Source: CAD feature listing. Evaluate the final solid. Frame: model axes, mm. Give positions to 0.01 mm unless a question says otherwise; leave off trailing zeros. Write each loop counter-clockwise with the first axis right and the second up, starting at its lowest first coordinate (ties: lowest second). Pieces come first, ordered by that corner, then holes.
```python
from build123d import *

# Parameters (mm, degrees)
SKETCH1_W           = 5
SKETCH1_H           = 28.000000001
SKETCH1_H_2         = 5
BOSS_EXTRUDE1_DEPTH = 5


with BuildPart() as part:
    # Sketch1 → Boss-Extrude1 (new body)
    with BuildSketch(Plane.XY):
        Polygon((331, 10), (323.5, 10), (323.5, 5), (318.5, 5), (318.5, 10), (2.5, 10), (2.5, 5), (-2.5, 5), (-2.5, 10), (-10, 10), (-10, 2.5), (-5, 2.5), (-5, -2.5), (-10, -2.5), (-10, -227.5), (-5, -227.5), (-5, -232.5), (-10, -232.5), (-10, -240), (-2.5, -240), (-2.5, -235), (2.5, -235), (2.5, -240), (318.5, -240), (318.5, -235), (323.5, -235), (323.5, -240), (331, -240), (331, -232.5), (326, -232.5), (326, -227.5), (331, -227.5), (331, -2.5), (326, -2.5), (326, 2.5), (331, 2.5), align=None)
        with Locations((-5.5, -128.600000001)):
            Rectangle(SKETCH1_W, SKETCH1_H, mode=Mode.SUBTRACT)
        with Locations((326.5, -128.600000001)):
            Rectangle(SKETCH1_W, SKETCH1_H, mode=Mode.SUBTRACT)
        with Locations((313.5, 0)):
            Rectangle(SKETCH1_W, SKETCH1_H_2, mode=Mode.SUBTRACT)
        with Locations((321, -7.5)):
            Rectangle(SKETCH1_W, SKETCH1_H_2, mode=Mode.SUBTRACT)
        with Locations((0, -7.5)):
            Rectangle(SKETCH1_W, SKETCH1_H_2, mode=Mode.SUBTRACT)
        with Locations((7.5, 0)):
            Rectangle(SKETCH1_W, SKETCH1_H_2, mode=Mode.SUBTRACT)
        with Locations((160.5, -122.5)):
            Rectangle(SKETCH1_W, SKETCH1_H_2, mode=Mode.SUBTRACT)
        with Locations((168, -115)):
            Rectangle(SKETCH1_W, SKETCH1_H_2, mode=Mode.SUBTRACT)
        with Locations((153, -115)):
            Rectangle(SKETCH1_W, SKETCH1_H_2, mode=Mode.SUBTRACT)
        with Locations((160.5, -107.5)):
            Rectangle(SKETCH1_W, SKETCH1_H_2, mode=Mode.SUBTRACT)
        with Locations((7.5, -230)):
            Rectangle(SKETCH1_W, SKETCH1_H_2, mode=Mode.SUBTRACT)
        with Locations((0, -222.5)):
            Rectangle(SKETCH1_W, SKETCH1_H_2, mode=Mode.SUBTRACT)
        with Locations((321, -222.5)):
            Rectangle(SKETCH1_W, SKETCH1_H_2, mode=Mode.SUBTRACT)
        with Locations((313.5, -230)):
            Rectangle(SKETCH1_W, SKETCH1_H_2, mode=Mode.SUBTRACT)
    extrude(amount=BOSS_EXTRUDE1_DEPTH)


solid = part.part
```
1. Line query: probe 1 along X at (y, z) = (-136, 0.2); probe 2 along X at (y, z) = (-221, 1.55); probe 3 along X at (y, z) = (-124, 3.6). Output: solid intervals per line, ascending.
2. Pin query (flat end, axial travel): P1, Ø2.5, axis at y = 0.5, z = 1.5, coming from the +X side; P2, Ø2.5, axis at y = -230.5, z = 3.5, coming from the -X side. Return the tip coordinate at first contact, or that it passes through.
3. Section query A-A (y = -137.5). Return loops of the section in (x, z), plus the area to 4 significant figures.
The answers:
1. probe 1: x = -10 to -8, -3 to 324, 329 to 331
1. probe 2: x = -10 to -2.5, 2.5 to 318.5, 323.5 to 331
1. probe 3: x = -10 to -8, -3 to 158, 163 to 324, 329 to 331
2. P1: stops at x = 326
2. P2: stops at x = -5
3. outline: (-10, 0) - (-8, 0) - (-8, 5) - (-10, 5) - close; (-3, 0) - (324, 0) - (324, 5) - (-3, 5) - close; (329, 0) - (331, 0) - (331, 5) - (329, 5) - close
3. area: 1,655 mm2
